from build123d import *

# Parameters (mm, degrees)
ESBO_O1_W                = 24
ESBO_O1_H                = 10
RESSALTO_EXTRUS_O1_DEPTH = 2
ESBO_O2_R                = 1.75
CORTE_EXTRUS_O1_DEPTH    = 14.601470509
FILETE1_R                = 2


with BuildPart() as part:
    # Esboço1 → Ressalto-extrusão1 (new, symmetric)
    with BuildSketch(Plane(origin=(0, 0, 0), x_dir=(1, 0, 0), z_dir=(0, 1, 0))):
        Rectangle(ESBO_O1_W, ESBO_O1_H)
    extrude(amount=RESSALTO_EXTRUS_O1_DEPTH, both=True)

    # Esboço2 → Corte-extrusão1 (cut, through all)
    with BuildSketch(Plane(origin=(0, 2, 0), x_dir=(1, 0, 0), z_dir=(0, 1, 0))):
        with Locations(Location((-9, 0, 0), (0, 0, 270))):
            Circle(ESBO_O2_R)
    corte_extrus_o1 = extrude(amount=-CORTE_EXTRUS_O1_DEPTH, mode=Mode.SUBTRACT)

    # Espelhar1: Corte-extrusão1 across plane
    add(corte_extrus_o1.mirror(Plane(origin=(0, 0, 0), x_dir=(0, 0, 1), z_dir=(1, 0, 0))), mode=Mode.SUBTRACT)

    # Filete1
    filete1_edges = [part.edges().sort_by_distance(p)[0] for p in [
        (12, 0, 5),
        (-12, 0, 5),
        (-12, 0, -5),
        (12, 0, -5),
    ]]
    fillet(filete1_edges, radius=FILETE1_R)


solid = part.part
Work out the finished part from the listing and answer in its coordinate system (mm). Coordinates: 2 decimals unless noted, no trailing zeros. Write each loop counter-clockwise with the first axis right and the second up, starting at its lowest first coordinate (ties: lowest second). Pieces come first, ordered by that corner, then holes.
1. For a pull along Z with two mould halves and no side action, classify faces 1 (the cylindrical face through (-7.265, 0.028, -0.228)), 2 (the flat face through (0, 0, -5)), 3 (the flat face through (0, 0, 5)) as +Z half, -Z half, draft (parallel to the pull), parting line (faces both ways), or undercut.
Results list:
face 1: undercut
face 2: -Z half
face 3: +Z half
2. A flat-ended cylindrical pin translates along its axis: pin 1 (2 mm diameter, centred on x = 9, z = 0, fed in from +Y). Find the tip coordinate at first contact, or state that the pin passes through.
Results list:
pin 1: passes through
3. Consider line 1 along X through (y, z) = (-0.95, 0); line 2 along X through (y, z) = (-0.95, -1); line 3 along Z through (x, y) = (8.5, 0.6). Determine where each line is inside the solid, lowest interval first.
Results list:
line 1: x = -12 to -10.75, -7.25 to 7.25, 10.75 to 12
line 2: x = -12 to -10.44, -7.56 to 7.56, 10.44 to 12
line 3: z = -5 to -1.68, 1.68 to 5
4. The part is cut by section C-C, the plane y = -0.45. Write down the section's boundary in (x, z).
Results list:
outline: (-12, -3) arc R2 ccw to (-10, -5) - (10, -5) arc R2 ccw to (12, -3) - (12, 3) arc R2 ccw to (10, 5) - (-10, 5) arc R2 ccw to (-12, 3) - close; hole circle Ø3.5 at (-9, 0); hole circle Ø3.5 at (9, 0)
5. The part is cut by section D-D, the plane z = 1. Write down the section's boundary in (x, y).
Results list:
outline: (-12, -2) - (-10.44, -2) - (-10.44, 2) - (-12, 2) - close; (-7.56, -2) - (7.56, -2) - (7.56, 2) - (-7.56, 2) - close; (10.44, -2) - (12, -2) - (12, 2) - (10.44, 2) - close
6. The part is cut by section A-A, the plane z = 0. Write down the section's boundary in (x, y).
Results list:
outline: (-12, -2) - (-10.75, -2) - (-10.75, 2) - (-12, 2) - close; (-7.25, -2) - (7.25, -2) - (7.25, 2) - (-7.25, 2) - close; (10.75, -2) - (12, -2) - (12, 2) - (10.75, 2) - close
7. The part is cut by section B-B, the plane x = 9. Write down the section's boundary in (y, z), and give its area (3 significant figures).
Results list:
outline: (-2, -5) - (2, -5) - (2, -1.75) - (-2, -1.75) - close; (-2, 1.75) - (2, 1.75) - (2, 5) - (-2, 5) - close
area: 26.0 mm2
